```python
from build123d import *

# Parameters (mm, degrees)
SKETCH1_R           = 15.5
BOSS_EXTRUDE1_DEPTH = 56
SKETCH4_R           = 25
BOSS_EXTRUDE2_DEPTH = 5
SKETCH5_R           = 10
CUT_EXTRUDE1_DEPTH  = 71.505318948
CUT_EXTRUDE2_DEPTH  = 4


with BuildPart() as part:
    # Sketch1 → Boss-Extrude1 (new body)
    with BuildSketch(Plane.XY):
        Circle(SKETCH1_R)
    extrude(amount=BOSS_EXTRUDE1_DEPTH)

    # Sketch4 → Boss-Extrude2 (add)
    with BuildSketch(Plane(origin=(0, 0, 0), x_dir=(-1, 0, 0), z_dir=(0, 0, -1))):
        Circle(SKETCH4_R)
    extrude(amount=BOSS_EXTRUDE2_DEPTH)

    # Sketch5 → Cut-Extrude1 (cut, through all)
    with BuildSketch(Plane.XY.offset(56)):
        Circle(SKETCH5_R)
    extrude(amount=-CUT_EXTRUDE1_DEPTH, mode=Mode.SUBTRACT)

    # Sketch6 → Cut-Extrude2 (cut, symmetric)
    with BuildSketch(Plane(origin=(0, 0, 0), x_dir=(1, 0, 0), z_dir=(0, 1, 0))):
        Polygon((12.5, -53.5), (10, -56), (15.5, -56), (15.5, -43), (12.5, -43), (11.5, -44), (11.5, -46), (12.5, -47), align=None)
    cut_extrude2 = extrude(amount=CUT_EXTRUDE2_DEPTH, both=True, mode=Mode.SUBTRACT)

    # Mirror1: Cut-Extrude2 across plane
    add(cut_extrude2.mirror(Plane(origin=(0, 0, 0), x_dir=(0, 0, 1), z_dir=(1, 0, 0))), mode=Mode.SUBTRACT)


solid = part.part
```
Can you work these out from the model? Positions are in its coordinate system, mm. A direction names the side the tool comes from. Round coordinates to 2 decimals unless told otherwise and drop trailing zeros. Loops run counter-clockwise (first coordinate to the right, second up) from the corner with the lowest first, then second, coordinate; pieces in that order, holes last. Notation, with made-up numbers: M 2.25,60.5 L 12.25,60.5 A23 ccw 12.25,89.5 Z; hole C -16.75,34 d5. An arc over 180 degrees is marked long. Answer as a JSON object with one key per item and string values. Group by question number.
Q1. Will these pins go through, and if not, where does the flat tip stop? pin 1 (4 mm diameter, centred on y = -8.5, z = 46, fed in from -X); pin 2 (1.5 mm diameter, centred on x = 12, z = 47.5, fed in from -Y); pin 3 (4 mm diameter, centred on x = -12, z = 47, fed in from +Y).
Q2. We'd pull the mould along Y, two halves only. Please class faces 5 (the flat face through (0, -11, -5)), 6 (the flat face through (-11.5, 0, 45)), 7 (the flat face through (14, 4, 49)), 8 (the cylindrical face through (14.784, 4.656, 27.608)): +Y half, -Y half, draft (parallel to the pull), parting line (faces both ways), or undercut.
Q3. Please list where these lines run through material, in increasing order: L1, parallel to Y at x = 0, z = 21; L2, parallel to Z at x = -20, y = 6; L3, parallel to X at y = -1.5, z = 51.5.
Q4. Imagine slicing it at D-D, the plane x = -5. Please give me the cut outline in (y, z).
Q5. Imagine slicing it at A-A, the plane x = 0. Please give me the cut outline in (y, z), then the cut area to 3 significant figures.
Q6. Imagine slicing it at B-B, the plane z = 48.5. Please give me the cut outline in (x, y), then the cut area to 3 significant figures.
Q7. On a 3-axis mill with a long thin cutter (end or side, diameter ignored), from which of +Z, -Z, +X, -X, +Y, -Y can I reach the whole of each face in a straight line? I mean faces 1 (the flat face through (-11, 0, 55)), 2 (the flat face through (11.5, 0, 45)), 3 (the flat face through (11.5, -10.8, 0)), 4 (the flat face through (12.5, 0, 50)). Say none if no direction works.
Q8. Imagine slicing it at C-C, the plane y = -13.5. Please give me the cut outline in (x, z).
Findings:
{
 "1": {"pin 1": "stops at x = -14.07", "pin 2": "stops at y = -10.66", "pin 3": "stops at y = 11.84"},
 "2": {"face 5": "draft", "face 6": "undercut", "face 7": "undercut", "face 8": "parting line"},
 "3": {"L1": "y = -15.5 to -10, 10 to 15.5", "L2": "z = -5 to 0", "L3": "x = -12.5 to -9.89, 9.89 to 12.5"},
 "4": {"outline": "M -24.49,-5 L -8.66,-5 L -8.66,56 L -14.67,56 L -14.67,0 L -24.49,0 Z; M 8.66,-5 L 24.49,-5 L 24.49,0 L 14.67,0 L 14.67,56 L 8.66,56 Z"},
 "5": {"outline": "M -25,-5 L -10,-5 L -10,56 L -15.5,56 L -15.5,0 L -25,0 Z; M 10,-5 L 25,-5 L 25,0 L 15.5,0 L 15.5,56 L 10,56 Z", "area": "766 mm2"},
 "6": {"outline": "M -14.97,-4 A15.5 ccw 14.97,-4 L 12.5,-4 L 12.5,4 L 14.97,4 A15.5 ccw -14.97,4 L -12.5,4 L -12.5,-4 Z; hole C 0,0 d20", "area": "395 mm2"},
 "7": {"face 1": "+Z, -X", "face 2": "+X", "face 3": "+Z", "face 4": "+Z, +X"},
 "8": {"outline": "M -21.04,-5 L 21.04,-5 L 21.04,0 L 7.62,0 L 7.62,56 L -7.62,56 L -7.62,0 L -21.04,0 Z"}
}
